Geometry: final body of the model. Coordinates: model frame, mm. A direction names the side the tool comes from. Give positions to 0.01 mm unless a question says otherwise; leave off trailing zeros. Order: outer loops, then holes, each group sorted by start corner. A loop starts at its lowest first (then second) coordinate and runs counter-clockwise, first axis right, second up. Notation, with made-up numbers: (-16, -12) -> (-3, -12) arc R29 ccw to (-3, 15) -> close; hole circle Ø11 at (82.5, 64). An arc over 180 degrees is marked (long way). Answer in a Markdown table with one row per item. Add a question column.
Q1. Cut plane A-A on y = 0. Return the cut outline in (x, z).
Q2. Contact query for flat-ended pins moving along their axis: P1, Ø6, axis at x = -17, y = 0, coming from the +Z side; P2, Ø4, axis at x = 20.5, y = 3.5, coming from the +Z side; P3, Ø3, axis at x = -6.5, z = -1, coming from the +Y side. Output: stop coordinate, or through.
Q3. Line query: line 1 along Y through (x, z) = (-25.25, 0); line 2 along X through (y, z) = (0, 0.75); line 3 along X through (y, z) = (5.5, -0.75). Output: solid intervals per line, ascending. Write a range as from..to.
Q4. Cut plane D-D on x = 6. Return the cut outline in (y, z), and give its area (3 significant figures).
Q5. Cut plane C-C on x = -25.25. Return the cut outline in (y, z), and give its area (3 significant figures).
Q6. Pull-direction query (Y, two-part tool) for faces 1 (the face through (-26.35, 0.05, 0.05)), 2 (the face through (0.42, 2.87, -2.64)), 3 (the face through (-30.25, 0, 0)); classes: +Y half, -Y half, draft (parallel to the pull), parting line (faces both ways), or undercut.
Q7. Cut plane B-B on z = -3.25. Return the cut outline in (x, y).
Q8. Set-up query: faces 4 (the face through (30.25, -3, -3)), 5 (the face through (31.73, 6.84, 0.9)). Return all of +Z, -Z, +X, -X, +Y, -Y with unobstructed straight access to the full face (end or side cutting, diameter ignored); none if empty.
from build123d import *

# Parameters (mm, degrees)
SKETCH2_3_R             = 1.1
CUT_EXTRUDE1_DEPTH      = 4.9
CUT_EXTRUDE1_DEPTH_BACK = 4.9
SKETCH3_R               = 6.9
BOSS_EXTRUDE1_DEPTH     = 3


with BuildPart() as part:
    # Sketch2 → Revolve2 (revolve)
    with BuildSketch(Plane.XY):
        with BuildLine():
            Line((30.25, 0), (-24.15, 0))
            ThreePointArc((-24.15, 0), (-25.25, -1.1), (-26.35, 0))
            Line((-26.35, 0), (-30.25, 0))
            Line((-30.25, 0), (-30.25, -3.9))
            Line((-30.25, -3.9), (30.25, -3.9))
            Line((30.25, -3.9), (30.25, 0))
        make_face()
    revolve(axis=Axis((-30.25, 0, 0), (1, 0, 0)))

    # Sketch2<3> → Cut-Extrude1 (cut, two sides)
    with BuildSketch(Plane.XY) as cut_extrude1_sk:
        with Locations((-25.25, 0)):
            Circle(SKETCH2_3_R)
    extrude(amount=CUT_EXTRUDE1_DEPTH, mode=Mode.SUBTRACT)
    extrude(cut_extrude1_sk.sketch, amount=-CUT_EXTRUDE1_DEPTH_BACK, mode=Mode.SUBTRACT)

    # Sketch3 → Boss-Extrude1 (add)
    with BuildSketch(Plane(origin=(30.25, 0, 0), x_dir=(0, 0, -1), z_dir=(1, 0, 0))):
        Circle(SKETCH3_R)
    extrude(amount=BOSS_EXTRUDE1_DEPTH)


solid = part.part
Completed:
| question | item | result |
|---|---|---|
| 1 | outline | (-30.25, -3.9) -> (-26.35, -3.9) -> (-26.35, 3.9) -> (-30.25, 3.9) -> close; (-24.15, -3.9) -> (30.25, -3.9) -> (30.25, -6.9) -> (33.25, -6.9) -> (33.25, 6.9) -> (30.25, 6.9) -> (30.25, 3.9) -> (-24.15, 3.9) -> close |
| 2 | P1 | stops at z = 3.9 |
| 2 | P2 | stops at z = 3.6 |
| 2 | P3 | stops at y = 3.9 |
| 3 | line 1 | y = -3.9..-1.1, 1.1..3.9 |
| 3 | line 2 | x = -30.25..-26.35, -24.15..33.25 |
| 3 | line 3 | x = 30.25..33.25 |
| 4 | outline | circle Ø7.8 at (0, 0) |
| 4 | area | 47.8 mm² |
| 5 | outline | (-1.1, -3.74) -> (-1.1, 3.74) arc R3.9 ccw to start; (1.1, -3.74) arc R3.9 ccw to (1.1, 3.74) -> close |
| 5 | area | 30.9 mm² |
| 6 | face 1 | undercut |
| 6 | face 2 | parting line |
| 6 | face 3 | draft |
| 7 | outline | (-30.25, -2.16) -> (30.25, -2.16) -> (30.25, -6.09) -> (33.25, -6.09) -> (33.25, 6.09) -> (30.25, 6.09) -> (30.25, 2.16) -> (-30.25, 2.16) -> close; hole circle Ø2.2 at (-25.25, 0) |
| 8 | face 4 | -X |
| 8 | face 5 | +X, -X |
